Source: CAD feature listing. Evaluate the final solid. Frame: model axes, mm. Round coordinates to 2 decimals unless told otherwise and drop trailing zeros. Write each loop counter-clockwise with the first axis right and the second up, starting at its lowest first coordinate (ties: lowest second). Pieces come first, ordered by that corner, then holes.
Autodesk Inventor part; units mm, degrees
ref_plane "作業平面1" through (0, 0, 0) normal (0, 0, 1) x (1, 0, 0)
ref_plane "YZ Plane" through (0, 0, 0) normal (1, 0, 0) x (0, 1, 0)
ref_plane "XZ Plane" through (0, 0, 0) normal (0, 1, 0) x (-1, 0, 0)
ref_plane "作業平面1" through (0, 0, 0) normal (0, 0, 1) x (1, 0, 0)
sketch "スケッチ1" plane through (0, 0, 0) normal (0, 0, 1) x (1, 0, 0)
  circle A0 centre (30.9729, -9.6966) radius 0.65
  circle A1 centre (27.8206, 6.7032) radius 0.65
  circle A2 centre (37.1456, -4.6077) radius 0.65
  circle A3 centre (23.6098, -6.2676) radius 0.65
  circle A4 centre (35.1836, 3.2742) radius 0.65
  circle A5 centre (21.6479, 1.6142) radius 0.65
  circle A6 centre (24.6258, 4.2902) radius 0.65
  circle A7 centre (34.1676, -7.2837) radius 0.65
  circle A8 centre (32.5077, 6.2521) radius 0.65
  circle A9 centre (26.2858, -9.2456) radius 0.65
  circle A10 centre (37.5966, 0.0794) radius 0.65
  circle A11 centre (21.1968, -3.0729) radius 0.65
  circle A12 centre (29.3967, -1.4967) radius 1.4
  circle A13 centre (29.3967, -1.4967) radius 10
  circle A14 centre (29.3967, -1.4967) radius 5
  circle A15 centre (42.1192, -16.9285) radius 1.25
  line L0 (29.3967, -1.4967) -> (34.1676, -7.2837)
  circle A16 centre (42.1192, -16.9285) radius 5
  line L1 (38.2612, -20.1091) -> (25.5388, -4.6773)
  line L2 (45.9771, -13.7479) -> (33.2547, 1.6839)
  circle A17 centre (29.3967, -1.4967) radius 11
  point P0 (0, 0)
  dimension "d0" = 10
  dimension "d1" = 2.5
  dimension "d2" = 20
  dimension "d3" = 10
  dimension "d4" = 22
extrude "押し出し1" add sketch "スケッチ1" along normal blind 3 contours A13 L2 A14 L1 | A13 L1 A17 L2 | L1 A14 L2 A13 | A13 L2 A17 L1 | A17 L2 A16 L1 | A16
properties part number "hornLink"
1) Section query A-A on x = 29.5. Return the cut outline in (y, z), then the cut area to 3 significant figures.
Taken from the geometry:
outline: (-12.5, 0) - (-6.5, 0) - (-6.5, 3) - (-12.5, 3) - close; (3.5, 0) - (9.5, 0) - (9.5, 3) - (3.5, 3) - close
area: 36.0 mm2
2) Material intervals for line 1 (Y direction, x = 29.5, z = 1.1); line 2 (X direction, y = -6, z = 1.6); line 3 (X direction, y = -0.5, z = 1.6), sorted ascending.
Taken from the geometry:
line 1: y = -12.5 to -6.5, 3.5 to 9.5
line 2: x = 19.36 to 23.02, 24.2 to 27.22, 31.57 to 39.59
line 3: x = 18.44 to 24.5, 34.3 to 37.3, 37.89 to 40.35
3) Section query B-B on y = -1. Return the cut outline in (x, z), then the cut area to 3 significant figures.
Taken from the geometry:
outline: (18.41, 0) - (24.42, 0) - (24.42, 3) - (18.41, 3) - close; (34.37, 0) - (40.39, 0) - (40.39, 3) - (34.37, 3) - close
area: 36.1 mm2
4) Pull-direction query (Y, two-part tool) for faces 1 (the face through (35.062, -16.228, 1.479)), 2 (the face through (30.832, -9.062, 1.479)), 3 (the face through (33, -6, 3)); classes: released by +Y, released by -Y, zero draft, split by the parting line, or undercut.
Taken from the geometry:
face 1: released by -Y
face 2: undercut
face 3: zero draft
5) Contact query for flat-ended pins moving along their axis: P1, Ø1.5, axis at x = 24.5, z = 2, coming from the +Y side; P2, Ø1, axis at y = -9.5, z = 1, coming from the -X side. Output: stop coordinate, or through.
Taken from the geometry:
P1: stops at y = 8.69
P2: stops at x = 21.35
6) Section query C-C on z = 0.6. State how many separate pieces and enclosed holes the cut face has, then the cut area to 3 significant figures.
Taken from the geometry:
separate pieces: 1
enclosed holes: 14
area: 414 mm2
